from build123d import *

# Parameters (mm, degrees)
SKETCH1_R           = 9
BOSS_EXTRUDE1_DEPTH = 25
SKETCH2_R           = 6
BOSS_EXTRUDE2_DEPTH = 40
CHAMFER1_SIZE       = 2


with BuildPart() as part:
    # Sketch1 → Boss-Extrude1 (new, symmetric)
    with BuildSketch(Plane(origin=(0, 0, 0), x_dir=(1, 0, 0), z_dir=(0, 1, 0))):
        with Locations(Location((0, 0, 0), (0, 0, 270))):
            Circle(SKETCH1_R)
    extrude(amount=BOSS_EXTRUDE1_DEPTH, both=True)

    # Sketch2 → Boss-Extrude2 (add, symmetric)
    with BuildSketch(Plane(origin=(0, 0, 0), x_dir=(1, 0, 0), z_dir=(0, 1, 0))):
        with Locations(Location((0, 0, 0), (0, 0, 270))):
            Circle(SKETCH2_R)
    extrude(amount=BOSS_EXTRUDE2_DEPTH, both=True)

    # Chamfer1
    chamfer1_edges = [part.edges().sort_by_distance(p)[0] for p in [
        (0, -40, -6),
        (0, 40, -6),
    ]]
    chamfer(chamfer1_edges, length=CHAMFER1_SIZE)


solid = part.part
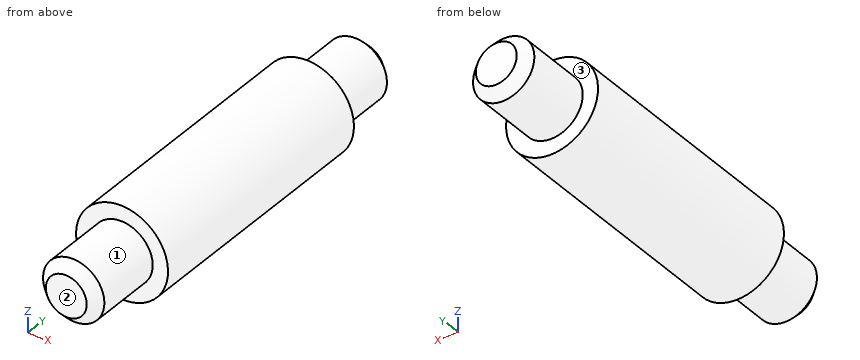
Input: part model. Units: mm. Frame: model coordinates. Face numbers are marked on the shaded views. A direction names the side the tool comes from. Give positions to 0.01 mm unless a question says otherwise; leave off trailing zeros. Order: outer loops, then holes, each group sorted by start corner. A loop starts at its lowest first (then second) coordinate and runs counter-clockwise, first axis right, second up. Notation, with made-up numbers: (41.5, 49) - (82.5, 49) arc R3 cw to (82.5, 53) - close; hole circle Ø2 at (-16, 1). An arc over 180 degrees is marked (long way). Answer as a JSON object with one key per item and string values. Group by question number.
Q1. Cut plane D-D, the plane y = -30. Output: boundary loops of the cut face in (x, z).
Q2. Cut plane C-C, the plane y = -7. Output: boundary loops of the cut face in (x, z), then the cut area to 3 significant figures.
Q3. Cut plane B-B, the plane z = 0. Output: boundary loops of the cut face in (x, y), then the cut area to 3 significant figures.
Q4. Line query: probe 1 along Z at (x, y) = (0.5, -22); probe 2 along Y at (x, z) = (-5.5, -2.5); probe 3 along X at (y, z) = (32.5, 0.25). Output: solid intervals per line, ascending.
Q5. Cut plane A-A, the plane x = 0. Output: boundary loops of the cut face in (y, z), then the cut area to 3 significant figures.
Q6. First-contact query: pin 1 Ø4 at (x, y) = (4, -17.5) entering from -Z; pin 2 Ø10 at (x, y) = (-5.5, 26) entering from -Z; pin 3 Ø1 at (x, z) = (-2.5, 5) entering from -Y. Flat tips, straight axial feed; report the tip coordinate or a pass-through.
Q7. Set-up query: the marked faces 1, 2 and 3. Return all of +Z, -Z, +X, -X, +Y, -Y with unobstructed straight access to the full face (end or side cutting, diameter ignored); none if empty.
Results:
{
 "1": {"outline": "circle Ø12 at (0, 0)"},
 "2": {"outline": "circle Ø18 at (0, 0)", "area": "254 mm^2"},
 "3": {"outline": "(-9, -25) - (-6, -25) - (-6, -38) - (-4, -40) - (4, -40) - (6, -38) - (6, -25) - (9, -25) - (9, 25) - (6, 25) - (6, 38) - (4, 40) - (-4, 40) - (-6, 38) - (-6, 25) - (-9, 25) - close", "area": "1,250 mm^2"},
 "4": {"probe 1": "-8.99 to 8.99", "probe 2": "-25 to 25", "probe 3": "-5.99 to 5.99"},
 "5": {"outline": "(-40, -4) - (-38, -6) - (-25, -6) - (-25, -9) - (25, -9) - (25, -6) - (38, -6) - (40, -4) - (40, 4) - (38, 6) - (25, 6) - (25, 9) - (-25, 9) - (-25, 6) - (-38, 6) - (-40, 4) - close", "area": "1,250 mm^2"},
 "6": {"pin 1": "z = -8.77", "pin 2": "z = -8.98", "pin 3": "y = -38.91"},
 "7": {"face 1": "-Y", "face 2": "+Z, -Z, +X, -X, -Y", "face 3": "+Y"}
}
